Autodesk Inventor part; units mm, degrees
ref_plane "YZ Plane" through (0, 0, 0) normal (1, 0, 0) x (0, 1, 0)
ref_plane "XZ Plane" through (0, 0, 0) normal (0, 1, 0) x (-1, 0, 0)
ref_plane "XY Plane" through (0, 0, 0) normal (0, 0, 1) x (1, 0, 0)
sketch "Sketch1" plane through (0, 0, 0) normal (0, 0, 1) x (1, 0, 0)
  line L0 (-5.0801, 28.6808) -> (14.9199, 28.6808)
  line L1 (14.9199, 28.6808) -> (14.9199, -8.3192)
  line L2 (14.9199, -8.3192) -> (-5.0801, -8.3192)
  line L3 (-5.0801, -8.3192) -> (-5.0801, 28.6808)
  line L4 (-5.0801, 28.6808) -> (-2.0801, 28.6808)
  line L5 (-2.0801, 28.6808) -> (-2.0801, -8.3192)
  line L6 (-2.0801, -8.3192) -> (-5.0801, -8.3192)
  line L7 (-5.0801, -8.3192) -> (-5.0801, 28.6808)
  point P0 (0, 0)
  dimension "d0" = 3
  dimension "d1" = 17
  dimension "d12" = 37
extrude "Extrusion1" add sketch "Sketch1" along normal blind 3
extrude "Extrusion2" add sketch "Sketch1" against normal blind 6 contours L0 L5 L2 L3
sketch "Sketch2" plane through (-5.0801, -8.3192, 3) normal (-1, 0, 0) x (0, 0, 1)
  circle A0 centre (-5, 4) radius 1.9
  circle A1 centre (-5, 33) radius 1.9
  line L0 (-3, 0) -> (-3, 37)
  line L1 (-9, 0) -> (0, 0)
  line L2 (-9, 37) -> (0, 37)
  line L3 (-9, 0) -> (-9, 37)
  line L4 (0, 37) -> (0, 0)
  point P0 (-3, 8.3192)
  dimension "d6" = 3.8
  dimension "d7" = 3.8
  dimension "d10" = 4
  dimension "d11" = 4
  dimension "d17" = 4
  dimension "d18" = 4
  dimension "d19" = 5
extrude "Extrusion3" cut sketch "Sketch2" against normal blind 6 contours A0 | A1
fillet "Fillet1" radius 3 1 edges at (-2.0801, 10.1808, 0)
fillet "Fillet2" radius 2 4 edges at (-3.5801, 28.6808, -6) (-3.5801, -8.3192, -6) (14.9199, 28.6808, 1.5) (14.9199, -8.3192, 1.5)
sketch "Sketch3" plane through (0, 0, 3) normal (0, 0, 1) x (1, 0, 0)
  point P0 (0, 0)
properties part number "psu side brace"
Model file for the job. Use its own axes, mm. A direction names the side the tool comes from. Give positions to 0.01 mm unless a question says otherwise; leave off trailing zeros. Order: outer loops, then holes, each group sorted by start corner. A loop starts at its lowest first (then second) coordinate and runs counter-clockwise, first axis right, second up. Notation, with made-up numbers: (-19.75, -39) - (15.25, -39) arc R13 ccw to (15.25, -18) - close; hole circle Ø1 at (54, 32). An arc over 180 degrees is marked (long way). Return JSON: item names as keys, results as strings.
1) Cut at B-B, the plane z = -3.5. Give the cut face in (x, y).
Geometry says:
{"outline": "(-5.08, -8.32) - (-2.08, -8.32) - (-2.08, -5.49) - (-5.08, -5.49) - close; (-5.08, -3.15) - (-2.08, -3.15) - (-2.08, 23.51) - (-5.08, 23.51) - close; (-5.08, 25.85) - (-2.08, 25.85) - (-2.08, 28.68) - (-5.08, 28.68) - close"}
2) Cut at A-A, the plane y = -5. Give the cut face in (x, z).
Geometry says:
{"outline": "(-5.08, -6) - (-2.08, -6) - (-2.08, -3.77) - (-5.08, -3.77) - close; (-5.08, -0.23) - (-0.22, -0.23) arc R3 cw to (0.92, 0) - (14.92, 0) - (14.92, 3) - (-5.08, 3) - close"}
3) Cut at D-D, the plane x = -0.25. Give the cut face in (y, z).
Geometry says:
{"outline": "(-8.32, -0.24) - (-5.03, -0.24) arc R1.9 cw to (-3.61, -0.24) - (23.97, -0.24) arc R1.9 cw to (25.39, -0.24) - (28.68, -0.24) - (28.68, 3) - (-8.32, 3) - close"}
4) Flat gauge pins, fed straight in: P1, Ø5, axis at y = 24.68, z = -2, coming from the -X side; P2, Ø0.9, axis at y = 4.5, z = -4.5, coming from the +X side; P3, Ø11, axis at x = 10.5, y = 8, coming from the -Z side. Where does each tip first touch, or does it go through?
Geometry says:
{"P1": "x = -5.08", "P2": "x = -2.08", "P3": "z = 0"}
5) Pull direction Y, two halves, no side cores. Call faces 3 (the cylindrical face through (-3.082, 25.252, -0.188)), 4 (the cylindrical face through (14.32, -7.75, 1.52)), 5 (the cylindrical face through (14.35, 28.08, 1.52)), 6 (the flat face through (8, 10, 0)): pulls with the +Y half, pulls with the -Y half, needs draft (parallel to the pull), parting line crosses it, or undercut.
Geometry says:
{"face 3": "undercut", "face 4": "pulls with the -Y half", "face 5": "pulls with the +Y half", "face 6": "needs draft"}
6) Cut at C-C, the plane y = 20. Give the cut face in (x, z).
Geometry says:
{"outline": "(-5.08, -6) - (-2.08, -6) - (-2.08, -3) arc R3 cw to (0.92, 0) - (14.92, 0) - (14.92, 3) - (-5.08, 3) - close"}
7) Probe line 1 (Y direction, x = -3.6, z = -2); line 2 (Z direction, x = 2.5, y = 16); line 3 (X direction, y = -2, z = -4.25). List the from-to ranges inside material, lowest first. Write a range as from..to.
Geometry says:
{"line 1": "-8.32..-6.22, -2.42..22.78, 26.58..28.68", "line 2": "0..3", "line 3": "-5.08..-2.08"}
8) 3-axis set-ups, long thin cutter, end or side, ignore diameter. For faces 1 (the flat face through (-5.08, 10, -1)), 2 (the flat face through (-2.08, 10, -4)): which of +Z, -Z, +X, -X, +Y, -Y reach the whole face in a straight line?
Geometry says:
{"face 1": "+Z, -Z, -X, +Y, -Y", "face 2": "-Z, +X, +Y, -Y"}
